Job drawing, mm, ordinate dimensions from the low corner. One solid piece. Give positions to 0.01 mm unless a question says otherwise; leave off trailing zeros. Write each loop counter-clockwise with the first axis right and the second up, starting at its lowest first coordinate (ties: lowest second). Pieces come first, ordered by that corner, then holes. Notation, with made-up numbers: M 40.25,26.5 L 67.25,26.5 A21 cw 67.25,33.5 Z; hole C 1.25,-20 d7. An arc over 180 degrees is marked long. Use CSV: the item, a comma, the result in double quotes. Start each with the question number.
Item 1: Drill centre lines: line 1 (Y direction, x = 160, z = 5); line 2 (Y direction, x = 241.5, z = 25); line 3 (X direction, y = 81.5, z = 5). Where is each one in solid material? Low to high. Write a range as [from, to].
Item 2: Cut at B-B (x = 184). List the corners of the cut face in (y, z), then the cut area to 3 significant figures.
Item 3: Cut at C-C (z = 5.5). List the corners of the cut face in (x, y) (3 decimals), then the cut area to 3 significant figures.
Item 4: Cut at A-A (y = 273.5). List the corners of the cut face in (x, z), then the cut area to 3 significant figures.
Item 5: Pin check, flat tips, straight feed: pin 1 (12 mm diameter, centred on x = 240, z = 19, fed in from -Y); pin 2 (4 mm diameter, centred on x = 120.5, z = 24, fed in from -Y); pin 3 (5 mm diameter, centred on y = 209, z = 8, fed in from -X). Stop position of each tip, or through.
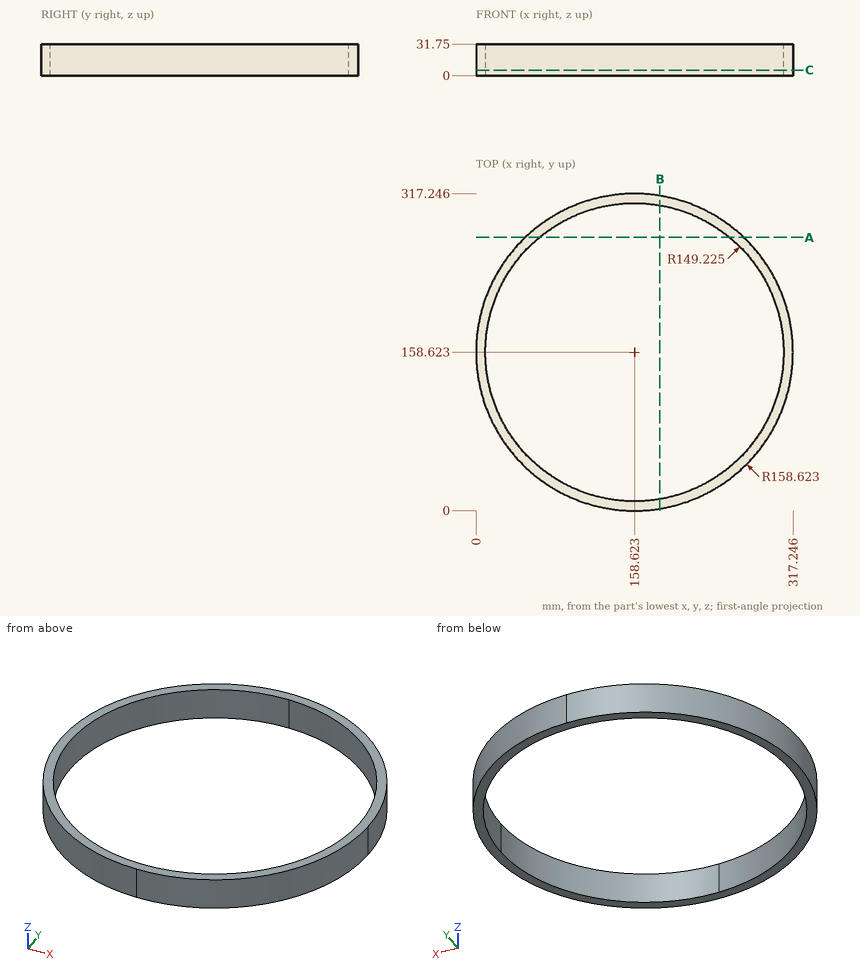
Worked answers:
1,line 1,"y = [0.01, 9.4], [307.84, 317.24]"
1,line 2,"y = [23.37, 34.53], [282.72, 293.87]"
1,line 3,"x = [20.01, 30.87], [286.37, 297.24]"
2,outline,"M 2.04,0 L 11.57,0 L 11.57,31.75 L 2.04,31.75 Z; M 305.67,0 L 315.2,0 L 315.2,31.75 L 305.67,31.75 Z"
2,area,"605 mm^2"
3,outline,"C 158.623,158.623 d317.246; hole M 158.623,9.398 A149.225 ccw 307.848,158.623 A149.225 ccw 158.623,307.848 A149.225 ccw Z"
3,area,"9,090 mm^2"
4,outline,"M 49.24,0 L 63.38,0 L 63.38,31.75 L 49.24,31.75 Z; M 253.87,0 L 268.01,0 L 268.01,31.75 L 253.87,31.75 Z"
4,area,"898 mm^2"
5,pin 1,"stops at y = 19.05"
5,pin 2,"stops at y = 4.17"
5,pin 3,"stops at x = 7.4"
